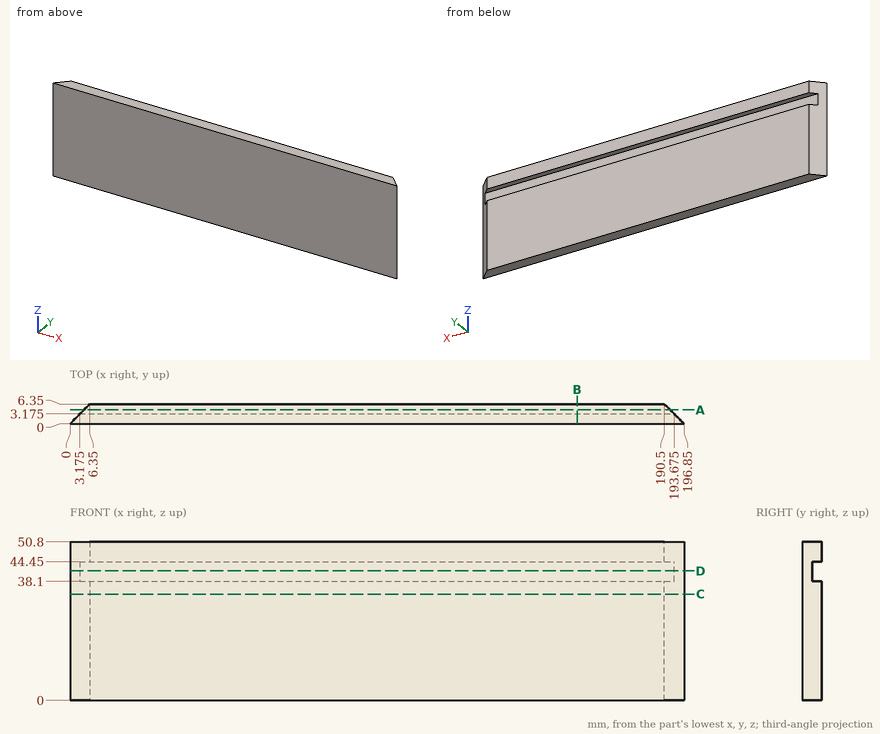
Input: dimensioned drawing with shaded views. Units: mm. Origin: part minimum x, y, z. Coordinates: 2 decimals unless noted, no trailing zeros. Write each loop counter-clockwise with the first axis right and the second up, starting at its lowest first coordinate (ties: lowest second). Pieces come first, ordered by that corner, then holes. Notation, with made-up numbers: M 38.25,18.5 L 95.25,18.5 A8 ccw 95.25,33.5 Z; hole C 58.5,-37.5 d1. An arc over 180 degrees is marked long. Use a Markdown table: item, result.
1) Section C-C, the plane z = 34. Output: boundary loops of the cut face in (x, y), then the cut area to 3 significant figures.
Conclusion:
| item | result |
|---|---|
| outline | M 0,0 L 196.85,0 L 190.5,6.35 L 6.35,6.35 Z |
| area | 1,210 mm^2 |
2) Section D-D, the plane z = 41.5. Output: boundary loops of the cut face in (x, y) (3 decimals), then the cut area to 3 significant figures.
Conclusion:
| item | result |
|---|---|
| outline | M 0,0 L 196.85,0 L 193.675,3.175 L 3.175,3.175 Z |
| area | 615 mm^2 |
3) First-contact query: pin 1 Ø2 at (y, z) = (4, 30) entering from -X; pin 2 Ø2 at (x, z) = (147, 43) entering from +Y (3 decimals); pin 3 Ø2 at (y, z) = (2.5, 8) entering from +X. Flat tips, straight axial feed; report the tip coordinate or a pass-through.
Conclusion:
| item | result |
|---|---|
| pin 1 | stops at x = 3 |
| pin 2 | stops at y = 3.175 |
| pin 3 | stops at x = 195.35 |
4) Ray query, L1, parallel to Z at x = 165.5, y = 6; L2, parallel to X at y = 1, z = 44; L3, parallel to X at y = 1.25, z = 36.5. Return the intervals inside material, ascending.
Conclusion:
| item | result |
|---|---|
| L1 | z = 0 to 38.1, 44.45 to 50.8 |
| L2 | x = 1 to 195.85 |
| L3 | x = 1.25 to 195.6 |
5) Section B-B, the plane x = 162.5. Output: boundary loops of the cut face in (y, z) (3 decimals).
Conclusion:
| item | result |
|---|---|
| outline | M 0,0 L 6.35,0 L 6.35,38.1 L 3.175,38.1 L 3.175,44.45 L 6.35,44.45 L 6.35,50.8 L 0,50.8 Z |
6) Section A-A, the plane y = 4.5. Output: boundary loops of the cut face in (x, z), then the cut area to 3 significant figures.
Conclusion:
| item | result |
|---|---|
| outline | M 4.5,0 L 192.35,0 L 192.35,38.1 L 4.5,38.1 Z; M 4.5,44.45 L 192.35,44.45 L 192.35,50.8 L 4.5,50.8 Z |
| area | 8,350 mm^2 |
